Source: CAD feature listing. Evaluate the final solid. Frame: model axes, mm. A direction names the side the tool comes from. Give positions to 0.01 mm unless a question says otherwise; leave off trailing zeros. Write each loop counter-clockwise with the first axis right and the second up, starting at its lowest first coordinate (ties: lowest second). Pieces come first, ordered by that corner, then holes. Notation, with made-up numbers: (-4, 88) -> (8, 88) arc R19 ccw to (8, 125) -> close; hole circle Ø1 at (82.5, 7.5). An arc over 180 degrees is marked (long way). Write item = value, one per line.
from build123d import *

# Parameters (mm, degrees)
SKETCH1_R                = 5
SKETCH1_R_2              = 2.5
BOSS_EXTRUDE1_DEPTH      = 4
BOSS_EXTRUDE1_DEPTH_BACK = 2
SKETCH2_W                = 2.5
SKETCH2_H                = 1
CUT_EXTRUDE1_DEPTH       = 6
CUT_EXTRUDE1_DEPTH_BACK  = 6
SKETCH3_R                = 5.75
SKETCH3_R_2              = 5
BOSS_EXTRUDE2_DEPTH      = 1
SKETCH5_R                = 5.75
SKETCH5_R_2              = 5
BOSS_EXTRUDE3_DEPTH      = 1


with BuildPart() as part:
    # Sketch1 → Boss-Extrude1 (new body, two sides)
    with BuildSketch(Plane(origin=(0, 0, 0), x_dir=(1, 0, 0), z_dir=(0, 1, 0))) as boss_extrude1_sk:
        Circle(SKETCH1_R)
        Circle(SKETCH1_R_2, mode=Mode.SUBTRACT)
    extrude(amount=BOSS_EXTRUDE1_DEPTH)
    extrude(boss_extrude1_sk.sketch, amount=-BOSS_EXTRUDE1_DEPTH_BACK)

    # Sketch2 → Cut-Extrude1 (cut, two sides)
    with BuildSketch(Plane.XY) as cut_extrude1_sk:
        Rectangle(SKETCH2_W, SKETCH2_H)
    extrude(amount=CUT_EXTRUDE1_DEPTH, mode=Mode.SUBTRACT)
    extrude(cut_extrude1_sk.sketch, amount=-CUT_EXTRUDE1_DEPTH_BACK, mode=Mode.SUBTRACT)

    # Sketch3 → Boss-Extrude2 (add)
    with BuildSketch(Plane.XZ.offset(2)):
        Circle(SKETCH3_R)
        Circle(SKETCH3_R_2, mode=Mode.SUBTRACT)
    extrude(amount=-BOSS_EXTRUDE2_DEPTH)

    # Sketch5 → Boss-Extrude3 (add)
    with BuildSketch(Plane(origin=(0, 1, 0), x_dir=(1, 0, 0), z_dir=(0, 1, 0))):
        Circle(SKETCH5_R)
        Circle(SKETCH5_R_2, mode=Mode.SUBTRACT)
    extrude(amount=BOSS_EXTRUDE3_DEPTH)


solid = part.part
(1) Access query for faces 4 (the face through (4.619, 0.014, 1.915)), 5 (the face through (-2, 2, -5)), 6 (the face through (1.25, 0, 3)). Directions: +Z, -Z, +X, -X, +Y, -Y. A direction counts if a zero-diameter tool reaches every point of the face in a straight line with its end or side. Return the directions, or none.
Values follow:
face_4 = none
face_5 = +Y
face_6 = +Z, -Z
(2) Section query D-D (x = -1.75). Return loops of the section in (y, z), plus the area to 3 significant figures.
Values follow:
outline = (-2, -5.48) -> (-1, -5.48) -> (-1, -4.68) -> (1, -4.68) -> (1, -5.48) -> (2, -5.48) -> (2, -4.68) -> (4, -4.68) -> (4, -1.79) -> (-2, -1.79) -> close; (-2, 1.79) -> (4, 1.79) -> (4, 4.68) -> (2, 4.68) -> (2, 5.48) -> (1, 5.48) -> (1, 4.68) -> (-1, 4.68) -> (-1, 5.48) -> (-2, 5.48) -> close
area = 38.0 mm2
(3) Material intervals for line 1 (X direction, y = 1.75, z = 0); line 2 (X direction, y = 3.7, z = 0); line 3 (Y direction, x = 2, z = -4.75), sorted ascending.
Values follow:
line_1 = -5.75 to -2.5, 2.5 to 5.75
line_2 = -5 to -2.5, 2.5 to 5
line_3 = -2 to -1, 1 to 2
(4) Section query A-A (x = 0). Return loops of the section in (y, z), plus the area to 3 significant figures.
Values follow:
outline = (-2, -5.75) -> (-1, -5.75) -> (-1, -5) -> (-0.5, -5) -> (-0.5, -2.5) -> (-2, -2.5) -> close; (-2, 2.5) -> (-0.5, 2.5) -> (-0.5, 5) -> (-1, 5) -> (-1, 5.75) -> (-2, 5.75) -> close; (0.5, -5) -> (1, -5) -> (1, -5.75) -> (2, -5.75) -> (2, -5) -> (4, -5) -> (4, -2.5) -> (0.5, -2.5) -> close; (0.5, 2.5) -> (4, 2.5) -> (4, 5) -> (2, 5) -> (2, 5.75) -> (1, 5.75) -> (1, 5) -> (0.5, 5) -> close
area = 28.0 mm2
(5) First-contact query: pin 1 (4.5 mm diameter, centred on x = 0, z = 0, fed in from -Y); pin 2 (0.5 mm diameter, centred on y = 0, z = -3.5, fed in from -X); pin 3 (1.1 mm diameter, centred on y = 0, z = -4, fed in from +X); pin 4 (1.1 mm diameter, centred on y = 0, z = 3.5, fed in from +X). Flat tips, straight axial feed; report the tip coordinate or a pass-through.
Values follow:
pin_1 = through
pin_2 = -3.8
pin_3 = 3.62
pin_4 = 4.04
(6) Section query B-B (y = -0.2). Return loops of the section in (x, z).
Values follow:
outline = (-1.25, -4.84) -> (-1.25, -2.17) arc R2.5 cw to (-1.25, 2.17) -> (-1.25, 4.84) arc R5 ccw to start; (1.25, -4.84) arc R5 ccw to (1.25, 4.84) -> (1.25, 2.17) arc R2.5 cw to (1.25, -2.17) -> close
(7) Section query C-C (z = 0). Return loops of the section in (x, y), plus the area to 3 significant figures.
Values follow:
outline = (-5.75, -2) -> (-2.5, -2) -> (-2.5, 4) -> (-5, 4) -> (-5, 2) -> (-5.75, 2) -> (-5.75, 1) -> (-5, 1) -> (-5, -1) -> (-5.75, -1) -> close; (2.5, -2) -> (5.75, -2) -> (5.75, -1) -> (5, -1) -> (5, 1) -> (5.75, 1) -> (5.75, 2) -> (5, 2) -> (5, 4) -> (2.5, 4) -> close
area = 33.0 mm2
(8) Pull-direction query (Y, two-part tool) for faces 1 (the face through (1.25, 0, -3)), 2 (the face through (-0.33, 1.04, -2.48)), 3 (the face through (2.5, -2, -1.2)); classes: pulls with the +Y half, pulls with the -Y half, needs draft (parallel to the pull), parting line crosses it, or undercut.
Values follow:
face_1 = undercut
face_2 = needs draft
face_3 = pulls with the -Y half
